Could you check a few things on this model? Use its own coordinates, in mm. Give positions to 0.01 mm unless a question says otherwise; leave off trailing zeros. Loops run counter-clockwise (first coordinate to the right, second up) from the corner with the lowest first, then second, coordinate; pieces in that order, holes last. Notation, with made-up numbers: (84, 45.25) - (116, 45.25) arc R16 ccw to (116, 58.25) - close; hole circle Ø9 at (40, 53). An arc over 180 degrees is marked (long way). Answer in a Markdown table with one row per item. Add a question column.
```python
from build123d import *

# Parameters (mm, degrees)
BODYSKE_R    = 1.25
BODY_DEPTH   = 1.75
MODLUGSKE_R  = 1.25
MODLUG_DEPTH = 1.75


with BuildPart() as part:
    # BodySke → Body (new body)
    with BuildSketch(Plane.XY):
        with BuildLine():
            Line((6.15473831, -21.381807602), (5.12564003, -17.806678924))
            ThreePointArc((5.12564003, -17.806678924), (6.26268227, -15.113739212), (9.13415023, -15.660969609))
            ThreePointArc((9.13415023, -15.660969609), (10.710697658, -16.474976548), (12.402371606, -15.939861288))
            ThreePointArc((12.402371606, -15.939861288), (0, 18.15), (-12.402371606, -15.939861288))
            ThreePointArc((-12.402371606, -15.939861288), (-10.710697658, -16.474976548), (-9.13415023, -15.660969609))
            ThreePointArc((-9.13415023, -15.660969609), (-6.26268227, -15.113739212), (-5.12564003, -17.806678924))
            Line((-5.12564003, -17.806678924), (-6.15473831, -21.381807602))
            ThreePointArc((-6.15473831, -21.381807602), (0, 22.25), (6.15473831, -21.381807602))
        make_face()
        with Locations((7.359918802, -17.163543347)):
            Circle(BODYSKE_R, mode=Mode.SUBTRACT)
        with Locations((-7.359918802, -17.163543347)):
            Circle(BODYSKE_R, mode=Mode.SUBTRACT)
    extrude(amount=-BODY_DEPTH)

    # ModLugSke → ModLug (add, through all)
    with BuildSketch(Plane.XY):
        with BuildLine():
            Line((6.15473831, -21.381807602), (4.550273009, -15.80783083))
            ThreePointArc((4.550273009, -15.80783083), (4.558712973, -15.732043553), (4.618125604, -15.684241005))
            ThreePointArc((4.618125604, -15.684241005), (6.723383791, -14.903644199), (8.701845472, -13.841979099))
            ThreePointArc((8.701845472, -13.841979099), (8.770273624, -13.827802373), (8.831276161, -13.861891696))
            ThreePointArc((8.831276161, -13.861891696), (11.5450024, -15.176170025), (14.345137247, -14.057741457))
            Line((14.345137247, -14.057741457), (15.89150871, -15.573132342))
            ThreePointArc((15.89150871, -15.573132342), (11.399317041, -19.108062984), (6.15473831, -21.381807602))
        make_face()
        with Locations((7.359918802, -17.163543347)):
            Circle(MODLUGSKE_R, mode=Mode.SUBTRACT)
        with BuildLine():
            Line((-6.15473831, -21.381807602), (-4.550273009, -15.80783083))
            ThreePointArc((-4.550273009, -15.80783083), (-4.558712973, -15.732043553), (-4.618125604, -15.684241005))
            ThreePointArc((-4.618125604, -15.684241005), (-6.723383791, -14.903644199), (-8.701845472, -13.841979099))
            ThreePointArc((-8.701845472, -13.841979099), (-8.770273624, -13.827802373), (-8.831276161, -13.861891696))
            ThreePointArc((-8.831276161, -13.861891696), (-11.5450024, -15.176170025), (-14.345137247, -14.057741457))
            Line((-14.345137247, -14.057741457), (-15.89150871, -15.573132342))
            ThreePointArc((-15.89150871, -15.573132342), (-11.399317041, -19.108062984), (-6.15473831, -21.381807602))
        make_face()
        with Locations((-7.359918802, -17.163543347)):
            Circle(MODLUGSKE_R, mode=Mode.SUBTRACT)
    extrude(amount=-MODLUG_DEPTH)


solid = part.part
```
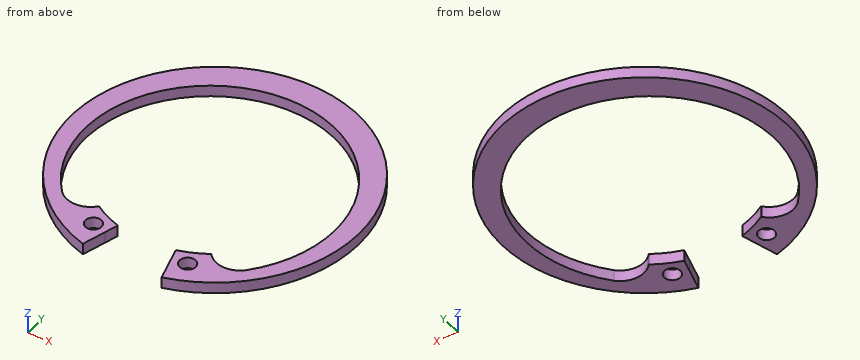
(1) I want a section at D-D on x = 0. Please give me the cut outline in (y, z), then the cut area to 4 significant figures.
(2) For pin 1 Ø3 at (x, y) = (7.36, -17.16) entering from +Z, with a flat end and sliding along its axis, tell me the tip position at first contact or that it passes through.
(3) I want a section at B-B on y = 7. Please give me the cut outline in (x, z).
(4) Please list where these lines run through material, in increasing order: line 1 (Y direction, x = -7.5, z = -0.65); line 2 (Y direction, x = 7, z = -1.65); line 3 (X direction, y = -17.5, z = -0.5).
(5) I want a section at C-C on z = -1.1. State how many separate pieces and enclosed holes the cut face has, then the cut area to 3 significant figures.
(6) I want a section at A-A on x = 11. Please give me the cut outline in (y, z).
Reported:
| question | item | result |
|---|---|---|
| 1 | outline | (18.15, -1.75) - (22.25, -1.75) - (22.25, 0) - (18.15, 0) - close |
| 1 | area | 7.175 mm² |
| 2 | pin 1 | z = 0 |
| 3 | outline | (-21.12, -1.75) - (-17.5, -1.75) - (-17.5, 0) - (-21.12, 0) - close; (17.5, -1.75) - (21.12, -1.75) - (21.12, 0) - (17.5, 0) - close |
| 4 | line 1 | -20.95 to -18.41, -15.92 to -14.53, 16.63 to 20.95 |
| 4 | line 2 | -21.12 to -18.36, -15.97 to -14.78, 16.84 to 21.12 |
| 4 | line 3 | -13.74 to -8.56, -6.16 to -5.04, 5.04 to 6.16, 8.56 to 13.74 |
| 5 | separate pieces | 1 |
| 5 | enclosed holes | 2 |
| 5 | area | 404 mm² |
| 6 | outline | (-19.34, -1.75) - (-15.12, -1.75) - (-15.12, 0) - (-19.34, 0) - close; (14.71, -1.75) - (19.34, -1.75) - (19.34, 0) - (14.71, 0) - close |
